Verification items for the finished model (mm, model axes). A direction names the side the tool comes from. Round coordinates to 2 decimals unless told otherwise and drop trailing zeros. Order: outer loops, then holes, each group sorted by start corner. A loop starts at its lowest first (then second) coordinate and runs counter-clockwise, first axis right, second up. Notation, with made-up numbers: M 32,66 L 85,66 A25 cw 85,96 Z; hole C 42,87.25 d6. An arc over 180 degrees is marked long. Return JSON: item names as keys, results as strings. Group by question number.
from build123d import *

# Parameters (mm, degrees)
SKETCH2_R            = 3
SKETCH2_R_2          = 8
BOSS_EXTRUDE1_DEPTH  = 37
M4_CLEARANCE_HOLE1_D = 3.6
CUT_EXTRUDE1_START   = -37
SKETCH2_3_R          = 3
CUT_EXTRUDE1_DEPTH   = 32


with BuildPart() as part:
    # Sketch2 → Boss-Extrude1 (new body)
    # profile 1 of 5: a face of its own
    with BuildSketch(Plane(origin=(0, 0, 0), x_dir=(0, 0, -1), z_dir=(1, 0, 0))):
        with BuildLine():
            Line((-24.16628289, -17.436478179), (-21.991350056, -15.506225289))
            ThreePointArc((-21.991350056, -15.506225289), (-17.756225289, -15.758649944), (-18.008649944, -19.993774711))
            Line((-18.008649944, -19.993774711), (-20.183582778, -21.924027601))
            ThreePointArc((-20.183582778, -21.924027601), (0, -29.8), (20.183582778, -21.924027601))
            Line((20.183582778, -21.924027601), (18.008649944, -19.993774711))
            ThreePointArc((18.008649944, -19.993774711), (17.756225289, -15.758649944), (21.991350056, -15.506225289))
            Line((21.991350056, -15.506225289), (24.16628289, -17.436478179))
            ThreePointArc((24.16628289, -17.436478179), (28.356615014, -9.162007692), (29.8, 0))
            ThreePointArc((29.8, 0), (-9.162007692, 28.356615014), (-24.16628289, -17.436478179))
        make_face()
        with Locations((-20, 2.25)):
            Circle(SKETCH2_R, mode=Mode.SUBTRACT)
        Circle(SKETCH2_R_2, mode=Mode.SUBTRACT)
        with Locations((20, 2.25)):
            Circle(SKETCH2_R, mode=Mode.SUBTRACT)
    # profile 2 of 5: a face of its own
    with BuildSketch(Plane(origin=(0, 0, 0), x_dir=(0, 0, -1), z_dir=(1, 0, 0))):
        with Locations((20, 2.25)):
            Circle(SKETCH2_R)
    # profile 3 of 5: a face of its own
    with BuildSketch(Plane(origin=(0, 0, 0), x_dir=(0, 0, -1), z_dir=(1, 0, 0))):
        with Locations((-20, 2.25)):
            Circle(SKETCH2_R)
    # profile 4 of 5: a face of its own
    with BuildSketch(Plane(origin=(0, 0, 0), x_dir=(0, 0, -1), z_dir=(1, 0, 0))):
        with BuildLine():
            ThreePointArc((20.183582778, -21.924027601), (22.28816213, -19.78074389), (24.16628289, -17.436478179))
            Line((24.16628289, -17.436478179), (21.991350056, -15.506225289))
            ThreePointArc((21.991350056, -15.506225289), (17.756225289, -15.758649944), (18.008649944, -19.993774711))
            Line((18.008649944, -19.993774711), (20.183582778, -21.924027601))
        make_face()
    # profile 5 of 5: a face of its own
    with BuildSketch(Plane(origin=(0, 0, 0), x_dir=(0, 0, -1), z_dir=(1, 0, 0))):
        with BuildLine():
            ThreePointArc((-18.008649944, -19.993774711), (-17.756225289, -15.758649944), (-21.991350056, -15.506225289))
            Line((-21.991350056, -15.506225289), (-24.16628289, -17.436478179))
            ThreePointArc((-24.16628289, -17.436478179), (-22.28816213, -19.78074389), (-20.183582778, -21.924027601))
            Line((-20.183582778, -21.924027601), (-18.008649944, -19.993774711))
        make_face()
    extrude(amount=-BOSS_EXTRUDE1_DEPTH)

    # M4 Clearance Hole1 (through all)
    with Locations(Plane.ZY.offset(37)):
        with Locations((-20, 2.25), (20, 2.25), (20, -17.75), (-20, -17.75)):
            Hole(M4_CLEARANCE_HOLE1_D / 2)

    # Sketch2<3> → Cut-Extrude1 (cut)
    with BuildSketch(Plane(origin=(0, 0, 0), x_dir=(0, 0, -1), z_dir=(1, 0, 0)).offset(CUT_EXTRUDE1_START)):
        with Locations((20, 2.25)):
            Circle(SKETCH2_3_R)
        with Locations((-20, 2.25)):
            Circle(SKETCH2_3_R)
        with BuildLine():
            ThreePointArc((-18.008649944, -19.993774711), (-17.756225289, -15.758649944), (-21.991350056, -15.506225289))
            Line((-21.991350056, -15.506225289), (-24.16628289, -17.436478179))
            ThreePointArc((-24.16628289, -17.436478179), (-22.28816213, -19.78074389), (-20.183582778, -21.924027601))
            Line((-20.183582778, -21.924027601), (-18.008649944, -19.993774711))
        make_face()
        with BuildLine():
            ThreePointArc((20.183582778, -21.924027601), (22.28816213, -19.78074389), (24.16628289, -17.436478179))
            Line((24.16628289, -17.436478179), (21.991350056, -15.506225289))
            ThreePointArc((21.991350056, -15.506225289), (17.756225289, -15.758649944), (18.008649944, -19.993774711))
            Line((18.008649944, -19.993774711), (20.183582778, -21.924027601))
        make_face()
    extrude(amount=CUT_EXTRUDE1_DEPTH, mode=Mode.SUBTRACT)


solid = part.part
1. Cross-section at C-C (y = -7). Enter the section's corners in (x, z), plus the area to 3 significant figures.
2. Cross-section at D-D (x = -3.5). Enter the section's corners in (y, z), plus the area to 3 significant figures.
3. Draft check along Z on faces 5 (the face through (0, -6, -6)), 6 (the face through (-5, 2, -22)), 7 (the face through (-21.224, -20.945, -19.081)). Enter one of: +Z half, -Z half, draft (parallel to the pull), parting line (faces both ways), or undercut.
4. Cross-section at A-A (z = 0). Enter the section's corners in (x, y).
5. Go/stop test with flat-tipped pins: pin 1 (5 mm diameter, centred on y = 1, z = 19.5, fed in from -X); pin 2 (4 mm diameter, centred on x = -22, y = 18, fed in from +Z); pin 3 (14.5 mm diameter, centred on y = 0, z = 0, fed in from +X); pin 4 (6 mm diameter, centred on x = -4.5, z = 0.5, fed in from +Y). Record where each tip stops, or that it passes through.
6. Cross-section at B-B (x = -30). Enter the section's corners in (y, z), plus the area to 3 significant figures.
7. Access from +Z, -Z, +X, -X, +Y, -Y to the whole of each face (thin tool, end or side, straight path). Record for faces 1 (the face through (-21.22, -20.97, 19.11)), 2 (the face through (-2.465, -15.965, -19.766)), 3 (the face through (-21.22, -15.81, 17.71)), 4 (the face through (-21.224, -16.458, 23.064)).
8. Thickness scan on line 1 along Y through (x, z) = (-3.25, 20); line 2 along Y through (x, z) = (-18.5, -20); line 3 along Z through (x, y) = (-1, -17). Record the ranges inside material, lowest first. Write a range as from..to.
Computed:
{
 "1": {"outline": "M -37,-28.97 L 0,-28.97 L 0,-3.87 L -37,-3.87 Z; M -37,3.87 L 0,3.87 L 0,28.97 L -37,28.97 Z", "area": "1,860 mm²"},
 "2": {"outline": "C 0,0 d59.6; hole C -17.75,-20 d3.6; hole C -17.75,20 d3.6; hole C 0,0 d16; hole C 2.25,-20 d3.6; hole C 2.25,20 d3.6", "area": "2,550 mm²"},
 "3": {"face 5": "draft", "face 6": "undercut", "face 7": "-Z half"},
 "4": {"outline": "M -37,-29.8 L 0,-29.8 L 0,-8 L -37,-8 Z; M -37,8 L 0,8 L 0,29.8 L -37,29.8 Z"},
 "5": {"pin 1": "stops at x = -37", "pin 2": "stops at z = 25.14", "pin 3": "passes through", "pin 4": "stops at y = 29.8"},
 "6": {"outline": "M -21.92,-20.18 L -19.99,-18.01 A3 cw -15.51,-21.99 L -17.44,-24.17 A29.8 ccw long -17.44,24.17 L -15.51,21.99 A3 cw -19.99,18.01 L -21.92,20.18 A29.8 ccw Z; hole C 0,0 d16; hole C 2.25,-20 d6; hole C 2.25,20 d6", "area": "2,470 mm²"},
 "7": {"face 1": "+Z, -X", "face 2": "+X, -X", "face 3": "-X", "face 4": "-X, -Y"},
 "8": {"line 1": "y = -22.09..-19.55, -15.95..0.45, 4.05..22.09", "line 2": "y = -22.09..-21.76, -14.75..-0.75, 5.25..22.09", "line 3": "z = -24.48..-21.64, -18.36..18.36, 21.64..24.48"}
}
